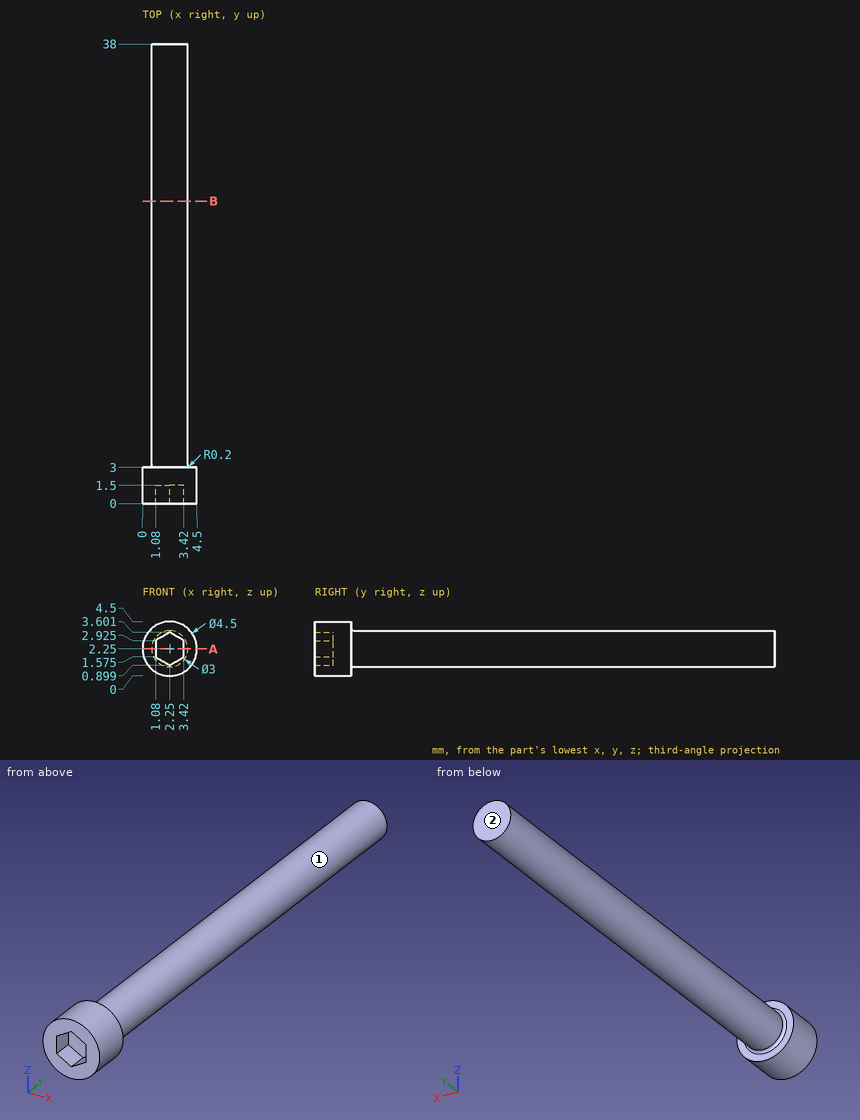
Geometry: see drawing. Coordinates: mm, zero at the bounding-box minimum. A direction names the side the tool comes from. Round coordinates to 2 decimals unless told otherwise and drop trailing zeros. Loops run counter-clockwise (first coordinate to the right, second up) from the corner with the lowest first, then second, coordinate; pieces in that order, holes last. Notation, with made-up numbers: (70, 80) - (127, 80) arc R36 cw to (127, 116) - close; hole circle Ø9 at (-37.75, 14). An arc over 180 degrees is marked (long way). One line per item, written item: value. Start each with the question number.
(1) Section B-B, the plane y = 25. Return loops of the section in (x, z).
(2) Ray query, line 1 (Y direction, x = 4.05, z = 1.2); line 2 (Z direction, x = 2.3, y = 36); line 3 (Y direction, x = 1.65, z = 2.75). Return the intervals inside material, ascending. Write a range as [from, to].
(3) Contact query for a flat-ended pin moving along its axis: P1, Ø1.5, axis at x = 2, y = 17, coming from the -Z side. Output: stop coordinate, or through.
(4) Section A-A, the plane z = 2.25. Return loops of the section in (x, y), plus the area to 3 significant figures.
(5) Access query for the marked faces 1 and 2. Directions: +Z, -Z, +X, -X, +Y, -Y. A direction counts if a zero-diameter tool reaches every point of the face in a straight line with its end or side. Return the directions, or none.
Results below:
1. outline: circle Ø3 at (2.25, 2.25)
2. line 1: [0, 3]
2. line 2: [0.75, 3.75]
2. line 3: [1.5, 38]
3. P1: z = 0.75
4. outline: (0, 0) - (1.08, 0) - (1.08, 1.5) - (3.42, 1.5) - (3.42, 0) - (4.5, 0) - (4.5, 3) - (3.95, 3) arc R0.2 cw to (3.75, 3.2) - (3.75, 38) - (0.75, 38) - (0.75, 3.2) arc R0.2 cw to (0.55, 3) - (0, 3) - close
4. area: 115 mm^2
5. face 1: +Y
5. face 2: +Z, -Z, +X, -X, +Y
